Source: CAD feature listing. Evaluate the final solid. Frame: model axes, mm. A direction names the side the tool comes from. Give positions to 0.01 mm unless a question says otherwise; leave off trailing zeros. Loops run counter-clockwise (first coordinate to the right, second up) from the corner with the lowest first, then second, coordinate; pieces in that order, holes last. Notation, with made-up numbers: (75, 42.25) - (94, 42.25) arc R18 ccw to (94, 76.25) - close; hole circle Ø11 at (21.5, -6). An arc over 180 degrees is marked (long way). Put each result on its own line as item: value.
```python
from build123d import *

# Parameters (mm, degrees)
CHAMFER1_SIZE           = 5
CUT_EXTRUDE1_REACH      = 304.159
CUT_EXTRUDE1_END_RADIUS = 65
SKETCH2_R               = 7.5


with BuildPart() as part:
    # Sketch1 → Revolve1 (revolve)
    with BuildSketch(Plane.XY, mode=Mode.PRIVATE) as revolve1_sk:
        with BuildLine():
            Line((80, 0), (120, 0))
            Line((120, 0), (120, 20))
            Line((120, 20), (90, 20))
            Line((90, 20), (61.860013717, 167.541531884))
            ThreePointArc((61.860013717, 167.541531884), (62.662860491, 168.934123661), (63.866098802, 170))
            Line((63.866098802, 170), (65, 170))
            Line((65, 170), (65, 250))
            Line((65, 250), (40, 250))
            Line((40, 250), (40, 170))
            Line((40, 170), (45, 170))
            ThreePointArc((45, 170), (46.885443724, 168.906865887), (48.126751856, 167.115499273))
            Line((48.126751856, 167.115499273), (80, 0))
        make_face()
    revolve(revolve1_sk.sketch.rotate(Axis((0, 126.434782609, 0), (0, -1, 0)), 90), axis=Axis((0, 126.434782609, 0), (0, -1, 0)))

    # Chamfer1
    chamfer1_edges = [part.edges().sort_by_distance(p)[0] for p in [
        (0, 250, -40),
    ]]
    chamfer(chamfer1_edges, length=CHAMFER1_SIZE)

    # Cut-Extrude1: up to this cylinder (the profile starts inside it)
    cut_extrude1_end = Plane(origin=(0, 210, 0), z_dir=(0, 1, 0)) * Cylinder(CUT_EXTRUDE1_END_RADIUS, 739.318, mode=Mode.PRIVATE)
    # Sketch2 → Cut-Extrude1 (cut, up to the surface)
    with BuildSketch(Plane.XY, mode=Mode.PRIVATE) as cut_extrude1_sk1:
        with Locations(Location((0, 210, 0), (0, 0, 180))):
            Circle(SKETCH2_R)
    cut_extrude1_tool1 = extrude(cut_extrude1_sk1.sketch, amount=CUT_EXTRUDE1_REACH, mode=Mode.PRIVATE) & cut_extrude1_end
    add(cut_extrude1_tool1.solids().sort_by_distance((0, 210, 0))[0], mode=Mode.SUBTRACT)


solid = part.part
```
1) Access query for faces 5 (the cylindrical face through (0.976, 202.564, 51.965)), 6 (the conical face through (23.27, 100.96, 56.11)), 7 (the flat face through (43, 170, -48)), 8 (the cylindrical face through (-19.52, 210.56, 62)). Directions: +Z, -Z, +X, -X, +Y, -Y. A direction counts if a zero-diameter tool reaches every point of the face in a straight line with its end or side. Return the directions, or none.
Check result:
face 5: +Z
face 6: -Y
face 7: none
face 8: +Y
2) Section query A-A, the plane z = 0. Output: boundary loops of the cut face in (x, y), plus the area to 3 significant figures.
Check result:
outline: (-120, 0) - (-80, 0) - (-48.13, 167.12) arc R5 cw to (-45, 170) - (-40, 170) - (-40, 245) - (-45, 250) - (-65, 250) - (-65, 170) - (-63.87, 170) arc R5 cw to (-61.86, 167.54) - (-90, 20) - (-120, 20) - close; (40, 170) - (45, 170) arc R5 cw to (48.13, 167.12) - (80, 0) - (120, 0) - (120, 20) - (90, 20) - (61.86, 167.54) arc R5 cw to (63.87, 170) - (65, 170) - (65, 250) - (45, 250) - (40, 245) - close
area: 9,810 mm²
3) Mould query, pull axis Z, two halves, no side actions, for faces 1 (the cylindrical face through (-101.184, 10.14, 64.511)), 2 (the cylindrical face through (-1.76, 206.98, -39.96)), 3 (the flat face through (26.5, 170, 30.2)), 4 (the flat face through (-44, 250, 14)). Classes: pulls with the +Z half, pulls with the -Z half, needs draft (parallel to the pull), parting line crosses it, or undercut.
Check result:
face 1: parting line crosses it
face 2: undercut
face 3: undercut
face 4: needs draft
4) Pin query (flat end, axial travel): P1, Ø1, axis at x = -27, y = 114.5, coming from the -Z side; P2, Ø10, axis at y = 42.5, z = -35.5, coming from the -X side; P3, Ø5, axis at y = 53.5, z = -64, coming from the -X side. Return the tip coordinate at first contact, or that it passes through.
Check result:
P1: z = -66.95
P2: x = -80.35
P3: x = -56.73
5) Section query B-B, the plane x = 0. State how many separate pieces and enclosed holes the cut face has, plus the area to 3 significant figures.
Check result:
separate pieces: 3
enclosed holes: 0
area: 9,430 mm²
6) Section query C-C, the plane y = 178. Output: boundary loops of the cut face in (x, z).
Check result:
outline: circle Ø130 at (0, 0); hole circle Ø80 at (0, 0)
7) Material intervals for line 1 along X through (y, z) = (207.5, 0); line 2 along Y through (x, z) = (-97, -35.5); line 3 along X through (y, z) = (210, 50), sorted ascending. Write a range as [from, to].
Check result:
line 1: [-65, -40], [40, 65]
line 2: [0, 20]
line 3: [-41.53, -7.5], [7.5, 41.53]
8) Section query D-D, the plane y = 210. Output: boundary loops of the cut face in (x, z), plus the area to 3 significant figures.
Check result:
outline: (-7.5, 39.29) - (-7.5, 64.57) arc R65 ccw (long way) to (7.5, 64.57) - (7.5, 39.29) arc R40 cw (long way) to start
area: 7,870 mm²
